Read the model definition and answer for the solid it produces. Units are mm, in the model's axes. A direction names the side the tool comes from. Coordinates: 2 decimals unless noted, no trailing zeros. Order: outer loops, then holes, each group sorted by start corner. A loop starts at its lowest first (then second) coordinate and runs counter-clockwise, first axis right, second up. Notation, with made-up numbers: M -4,63 L 17,63 A28 cw 17,89 Z; hole C 12.25,-28 d4. An arc over 180 degrees is marked long. Use a Markdown table: item, result. Add a question column.
1) Find section A-A on x = 48. Write down the section's boundary in (y, z) (3 decimals), plus the area to 3 significant figures.
2) Find section C-C on y = -30. Write down the section's boundary in (x, z), plus the area to 3 significant figures.
3) For faces 1 (the face through (303, -50.8, -85)), 2 (the face through (294, -25, -31.75)), 3 (the face through (294, -2.753, -13)), determine the directions among +Z, -Z, +X, -X, +Y, -Y from which every point of the face is accessible in a straight line to the end or side of a thin tool.
4) Find section B-B on z = -48. Write down the section's boundary in (x, y), plus the area to 3 significant figures.
5) Each of these flat-tipped pins is pushed along its axis until it touches: pin 1 Ø2 at (x, y) = (257, -38) entering from +Z; pin 2 Ø5 at (x, z) = (412, -70) entering from +Y; pin 3 Ø1 at (x, z) = (295, -30.5) entering from +Y. Where does it stop, or does it pass through?
6) Find the intervals of material crossed by probe 1 along Z at (x, y) = (378, -21.5); probe 2 along Y at (x, z) = (462, -75.5); probe 3 along Y at (x, z) = (554.5, -25), in increasing order. Write a range as [from, to].
from build123d import *

# Parameters (mm, degrees)
SKETCH1_W                    = 596.9
SKETCH1_H                    = 31.75
BASE_FLANGE1_DEPTH           = 2.75336
EDGE_FLANGE1_STRIP_W         = 17.36344
EDGE_FLANGE1_STRIP_H         = 2.75336
EDGE_FLANGE1_STRIP_CUT_DEPTH = 596.9
EDGE_FLANGE1_DEPTH           = 596.9
EDGE_FLANGE2_STRIP_W         = 17.36344
EDGE_FLANGE2_STRIP_H         = 2.75336
EDGE_FLANGE2_STRIP_CUT_DEPTH = 596.9
EDGE_FLANGE2_DEPTH           = 596.9
BREAK_CORNER1_START          = -50.8
BREAK_CORNER1_DEPTH          = 50.8


# Read off the part's stored shape, not the designer's step: Break-Corner1
# Sheet-metal steps are written as plain solids
with BuildPart() as part:
    # Sketch1 → Base-Flange1 (new body)
    with BuildSketch(Plane(origin=(0, 0, 0), x_dir=(1, 0, 0), z_dir=(0, 1, 0))):
        with Locations((298.45, 15.875)):
            Rectangle(SKETCH1_W, SKETCH1_H)
    extrude(amount=-BASE_FLANGE1_DEPTH)

    # Edge-Flange1 strip (across the edge) → Edge-Flange1 strip cut (cut)
    with BuildSketch(Plane(origin=(0, -2.75336, -31.75), x_dir=(0, 0, 1), z_dir=(1, 0, 0))):
        with Locations((-2.75336, -1.37668)):
            Rectangle(EDGE_FLANGE1_STRIP_W, EDGE_FLANGE1_STRIP_H)
    extrude(amount=EDGE_FLANGE1_STRIP_CUT_DEPTH, mode=Mode.SUBTRACT)

    # Edge-Flange1 section (across the edge) → Edge-Flange1 (add)
    with BuildSketch(Plane(origin=(0, -2.75336, -31.75), x_dir=(0, 0, 1), z_dir=(1, 0, 0))):
        with BuildLine():
            Line((0, 3.175), (0, 48.04664))
            Line((0, 48.04664), (2.75336, 48.04664))
            Line((2.75336, 48.04664), (2.75336, 3.175))
            ThreePointArc((2.75336, 3.175), (3.68329597, 0.92993597), (5.92836, 0))
            Line((5.92836, 0), (5.92836, -2.75336))
            ThreePointArc((5.92836, -2.75336), (1.736376443, -1.016983557), (0, 3.175))
        make_face()
    extrude(amount=EDGE_FLANGE1_DEPTH)

    # Edge-Flange2 strip (across the edge) → Edge-Flange2 strip cut (cut)
    with BuildSketch(Plane(origin=(596.9, -50.8, -31.75), x_dir=(0, 1, 0), z_dir=(-1, 0, 0))):
        with Locations((-2.75336, -1.37668)):
            Rectangle(EDGE_FLANGE2_STRIP_W, EDGE_FLANGE2_STRIP_H)
    extrude(amount=EDGE_FLANGE2_STRIP_CUT_DEPTH, mode=Mode.SUBTRACT)

    # Edge-Flange2 section (across the edge) → Edge-Flange2 (add)
    with BuildSketch(Plane(origin=(596.9, -50.8, -31.75), x_dir=(0, 1, 0), z_dir=(-1, 0, 0))):
        with BuildLine():
            Line((0, 3.175), (0, 104.775))
            Line((0, 104.775), (2.75336, 104.775))
            Line((2.75336, 104.775), (2.75336, 3.175))
            ThreePointArc((2.75336, 3.175), (3.68329597, 0.92993597), (5.92836, 0))
            Line((5.92836, 0), (5.92836, -2.75336))
            ThreePointArc((5.92836, -2.75336), (1.736376443, -1.016983557), (0, 3.175))
        make_face()
    extrude(amount=EDGE_FLANGE2_DEPTH)

    # Break-Corner1 outline → Break-Corner1 (cut)
    with BuildSketch(Plane(origin=(0, 0, 0), x_dir=(1, 0, 0), z_dir=(0, 1, 0)).offset(BREAK_CORNER1_START)):
        with BuildLine():
            Line((0, 0), (6.35, 0))
            ThreePointArc((6.35, 0), (1.859871939, 1.859871939), (0, 6.35))
            Line((0, 6.35), (0, 0))
        make_face()
        with BuildLine():
            ThreePointArc((596.9, 6.35), (595.040128061, 1.859871939), (590.55, 0))
            Line((590.55, 0), (596.9, 0))
            Line((596.9, 0), (596.9, 6.35))
        make_face()
        with BuildLine():
            ThreePointArc((0, 130.175), (1.859871939, 134.665128061), (6.35, 136.525))
            Line((6.35, 136.525), (0, 136.525))
            Line((0, 136.525), (0, 130.175))
        make_face()
        with BuildLine():
            ThreePointArc((590.55, 136.525), (595.040128061, 134.665128061), (596.9, 130.175))
            Line((596.9, 130.175), (596.9, 136.525))
            Line((596.9, 136.525), (590.55, 136.525))
        make_face()
    extrude(amount=BREAK_CORNER1_DEPTH, mode=Mode.SUBTRACT)


solid = part.part
Check result:
| question | item | result |
|---|---|---|
| 1 | outline | M -50.8,-136.525 L -48.047,-136.525 L -48.047,-34.925 A3.175 cw -44.872,-31.75 L -5.928,-31.75 A5.928 ccw 0,-25.822 L 0,0 L -2.753,0 L -2.753,-25.822 A3.175 cw -5.928,-28.997 L -44.872,-28.997 A5.928 ccw -50.8,-34.925 Z |
| 1 | area | 497 mm2 |
| 2 | outline | M 0,-31.75 L 596.9,-31.75 L 596.9,-29 L 0,-29 Z |
| 2 | area | 1,640 mm2 |
| 3 | face 1 | +Z, -Z, +X, -X, -Y |
| 3 | face 2 | -Z, +X, -X, +Y |
| 3 | face 3 | +Z, +X, -X, -Y |
| 4 | outline | M 0,-50.8 L 596.9,-50.8 L 596.9,-48.05 L 0,-48.05 Z |
| 4 | area | 1,640 mm2 |
| 5 | pin 1 | stops at z = -29 |
| 5 | pin 2 | stops at y = -48.05 |
| 5 | pin 3 | stops at y = -1.72 |
| 6 | probe 1 | z = [-31.75, -29] |
| 6 | probe 2 | y = [-50.8, -48.05] |
| 6 | probe 3 | y = [-2.75, 0] |
